from build123d import *

# Parameters (mm, degrees)
SALIENTE_EXTRUIR1_DEPTH = 2
CROQUIS2_R              = 1.5
SALIENTE_EXTRUIR4_DEPTH = 4.6


with BuildPart() as part:
    # Croquis1 → Saliente-Extruir1 (new body)
    with BuildSketch(Plane.XY):
        with BuildLine():
            Line((-1.249573298, 6.373923256), (-6.119309861, -2.067772542))
            ThreePointArc((-6.119309861, -2.067772542), (-6.118902164, -3.56753706), (-4.82, -4.317301652))
            Line((-4.82, -4.317301652), (4.92, -4.317301652))
            ThreePointArc((4.92, -4.317301652), (6.218902164, -3.56753706), (6.219309861, -2.067772542))
            Line((6.219309861, -2.067772542), (1.349573298, 6.373923256))
            ThreePointArc((1.349573298, 6.373923256), (0.05, 7.124546306), (-1.249573298, 6.373923256))
        make_face()
        with BuildLine():
            Line((-0.699721633, 4.324692275), (-4.070430344, -1.518015182))
            ThreePointArc((-4.070430344, -1.518015182), (-3.52108613, -2.067086511), (-3.32, -2.817301652))
            Line((-3.32, -2.817301652), (3.42, -2.817301652))
            ThreePointArc((3.42, -2.817301652), (3.62108613, -2.067086511), (4.170430344, -1.518015182))
            Line((4.170430344, -1.518015182), (0.799721633, 4.324692275))
            ThreePointArc((0.799721633, 4.324692275), (0.05, 4.12393805), (-0.699721633, 4.324692275))
        make_face(mode=Mode.SUBTRACT)
    extrude(amount=SALIENTE_EXTRUIR1_DEPTH)

    # Croquis2 → Saliente-Extruir4 (add)
    with BuildSketch(Plane.XY.offset(2)):
        with Locations((0.05, 5.624242178)):
            Circle(CROQUIS2_R)
        with Locations(Location((4.92, -2.817301652, 0), (0, 0, 180))):
            Circle(CROQUIS2_R)
        with Locations((-4.82, -2.817301652)):
            Circle(CROQUIS2_R)
    extrude(amount=SALIENTE_EXTRUIR4_DEPTH)


solid = part.part
The model under review builds one solid part; all positions refer to its coordinate system, in mm. A direction names the side the tool comes from. Round coordinates to 2 decimals unless told otherwise and drop trailing zeros. Loops run counter-clockwise (first coordinate to the right, second up) from the corner with the lowest first, then second, coordinate; pieces in that order, holes last. Notation, with made-up numbers: (35.25, -11) -> (63.25, -11) arc R29 ccw to (63.25, 11) -> close; hole circle Ø8 at (35, -12). An arc over 180 degrees is marked (long way). Write item = value, one per line. Start each with the question number.
Item 1: Insertion check: pin 1 (1.2 mm diameter, centred on x = 0.5, y = -4, fed in from +Z); pin 2 (1 mm diameter, centred on x = -1.5, z = 1, fed in from +Y); pin 3 (2 mm diameter, centred on x = -1.5, z = 2, fed in from +Y). Each pin has a flat end and moves straight along its axis. Give the tip position at first contact, or say it passes through.
Item 2: Take a section at B-B on y = 0.75. Give the boundary of the cut face in (x, z).
Item 3: Take a section at D-D on x = 5.5. Give the boundary of the cut face in (y, z), plus the area to 3 significant figures.
Item 4: For faces 4 (the flat face through (-2.361, 1.444, 0.986)), 5 (the cylindrical face through (-0.15, 7.11, 4.27)), 6 (the flat face through (0, -4, 2)), list the 3-axis set-ups (+Z, -Z, +X, -X, +Y, -Y) from which the entire face can be reached by the end or side of a thin tool; tool diameter is ignored.
Item 5: Mouldability with a two-part tool opening along Y and no side actions: class faces 1 (the cylindrical face through (0.061, 4.124, 0.986)), 2 (the flat face through (0, -4.317, 1)), 3 (the flat face through (-5, -3, 6.6)) as released by +Y, released by -Y, zero draft, split by the parting line, or undercut.
Item 6: To check wall thickness, follow L1, parallel to Z at x = -2.75, y = -3; L2, parallel to X at y = 3.5, z = 1.5; L3, parallel to X at y = 0.5, z = 0.5. State the ranges of each line that lie inside material, in increasing order.
Item 7: Take a section at A-A on z = 0.75. Give the boundary of the cut face in (x, y).
Result:
q1.pin_1 = 2
q1.pin_2 = 6.7
q1.pin_3 = 7.02
q2.outline = (-4.49, 0) -> (-2.76, 0) -> (-2.76, 2) -> (-4.49, 2) -> close; (2.86, 0) -> (4.59, 0) -> (4.59, 2) -> (2.86, 2) -> close
q3.outline = (-4.2, 0) -> (-0.82, 0) -> (-0.82, 2) -> (-1.43, 2) -> (-1.43, 6.6) -> (-4.2, 6.6) -> close
q3.area = 19.5 mm²
q4.face_4 = +Z, -Z
q4.face_5 = +Z
q4.face_6 = +Z, -Y
q5.face_1 = undercut
q5.face_2 = released by -Y
q5.face_3 = zero draft
q6.L1 = 0 to 2
q6.L2 = -2.91 to -1.18, 1.28 to 3.01
q6.L3 = -4.64 to -2.91, 3.01 to 4.74
q7.outline = (-6.12, -2.07) arc R1.5 ccw to (-4.82, -4.32) -> (4.92, -4.32) arc R1.5 ccw to (6.22, -2.07) -> (1.35, 6.37) arc R1.5 ccw to (-1.25, 6.37) -> close; hole (-4.07, -1.52) arc R1.5 cw to (-3.32, -2.82) -> (3.42, -2.82) arc R1.5 cw to (4.17, -1.52) -> (0.8, 4.32) arc R1.5 cw to (-0.7, 4.32) -> close
